Could you check a few things on this model? Use its own coordinates, in mm. Face numbers are marked on the shaded views. Coordinates: 2 decimals unless noted, no trailing zeros. Loops run counter-clockwise (first coordinate to the right, second up) from the corner with the lowest first, then second, coordinate; pieces in that order, holes last. Notation, with made-up numbers: (-21.5, 79) - (18.5, 79) arc R8 cw to (18.5, 89) - close; hole circle Ø5 at (88.25, 54.25). An arc over 180 degrees is marked (long way). Use CSV: the item, a comma, the result in double quotes.
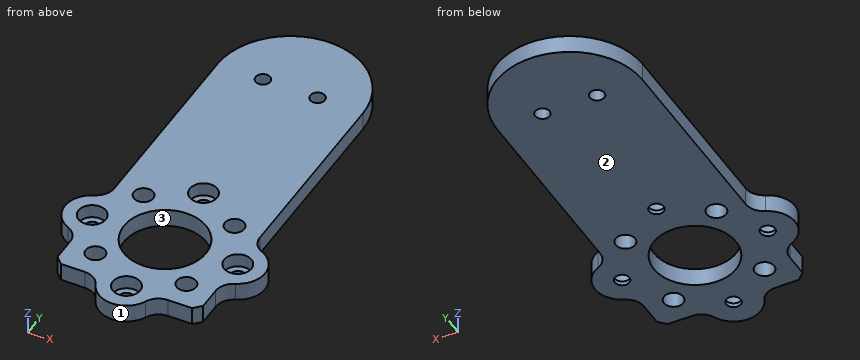
from build123d import *

# Parameters (mm, degrees)
SKETCH1_R                                       = 3.3782
SKETCH1_R_2                                     = 14.3129
BOSS_EXTRUDE1_DEPTH                             = 6.35
CBORE_FOR_10_SOCKET_HEAD_CAP_SCREW1_D           = 5.1054
CBORE_FOR_10_SOCKET_HEAD_CAP_SCREW1_CBORE_D     = 9.525
CBORE_FOR_10_SOCKET_HEAD_CAP_SCREW1_CBORE_DEPTH = 4.826
F_1_4_20_TAPPED_HOLE2_D                         = 5.1054
FILLET1_R                                       = 6.35
CHAMFER1_SIZE                                   = 2.54


with BuildPart() as part:
    # Sketch1 → Boss-Extrude1 (new body)
    with BuildSketch(Plane.XY):
        with BuildLine():
            Line((0, 0), (15.875, 0))
            ThreePointArc((15.875, 0), (25.4, -9.525), (34.925, 0))
            Line((34.925, 0), (50.8, 0))
            Line((50.8, 0), (50.8, 15.875))
            ThreePointArc((50.8, 15.875), (60.325, 25.4), (50.8, 34.925))
            Line((50.8, 34.925), (50.8, 107.95))
            ThreePointArc((50.8, 107.95), (25.4, 133.35), (0, 107.95))
            Line((0, 107.95), (0, 34.925))
            ThreePointArc((0, 34.925), (-9.525, 25.4), (0, 15.875))
            Line((0, 15.875), (0, 0))
        make_face()
        with Locations((41.275, 9.525)):
            Circle(SKETCH1_R, mode=Mode.SUBTRACT)
        with Locations((9.525, 9.525)):
            Circle(SKETCH1_R, mode=Mode.SUBTRACT)
        with Locations((9.525, 41.275)):
            Circle(SKETCH1_R, mode=Mode.SUBTRACT)
        with Locations((41.275, 41.275)):
            Circle(SKETCH1_R, mode=Mode.SUBTRACT)
        with Locations((25.4, 25.4)):
            Circle(SKETCH1_R_2, mode=Mode.SUBTRACT)
    extrude(amount=BOSS_EXTRUDE1_DEPTH)

    # CBORE for #10 Socket Head Cap Screw1 (through all)
    with Locations(Plane.XY.offset(6.35)):
        with Locations((0, 25.4), (50.8, 25.4), (25.4, 0), (25.4, 50.8)):
            CounterBoreHole(CBORE_FOR_10_SOCKET_HEAD_CAP_SCREW1_D / 2, CBORE_FOR_10_SOCKET_HEAD_CAP_SCREW1_CBORE_D / 2, CBORE_FOR_10_SOCKET_HEAD_CAP_SCREW1_CBORE_DEPTH)

    # 1/4-20 Tapped Hole2 (through all)
    with Locations(Plane(origin=(0, 0, 0), x_dir=(1, 0, 0), z_dir=(0, 0, -1))):
        with Locations((15.875, -107.95), (34.925, -107.95)):
            Hole(F_1_4_20_TAPPED_HOLE2_D / 2)

    # Fillet1
    fillet1_edges = [part.edges().sort_by_distance(p)[0] for p in [
        (0, 15.875, 3.175),
        (0, 34.925, 3.175),
        (50.8, 34.925, 3.175),
        (50.8, 15.875, 3.175),
        (34.925, 0, 3.175),
        (15.875, 0, 3.175),
    ]]
    fillet(fillet1_edges, radius=FILLET1_R)

    # Chamfer1
    chamfer1_edges = [part.edges().sort_by_distance(p)[0] for p in [
        (50.8, 0, 3.175),
        (0, 0, 3.175),
    ]]
    chamfer(chamfer1_edges, length=CHAMFER1_SIZE)


solid = part.part
(1) Thinking about a two-plate mould opening in X: for the marked faces 1, 2 and 3, which applies, +X half, -X half, draft (parallel to the pull), parting line (faces both ways), or undercut?
Computed:
face 1,"parting line"
face 2,"draft"
face 3,"undercut"
(2) Suppose I cut it at A-A (y = 25.4). State how many separate pieces and enclosed holes the cut face has, plus the area to 3 significant figures.
Computed:
separate pieces,"4"
enclosed holes,"0"
area,"154 mm²"
(3) Will these pins go through, and if not, where does the flat tip stop? pin 1 (1 mm diameter, centred on x = 49.5, z = 4, fed in from -Y); pin 2 (1 mm diameter, centred on x = 26.5, z = 2.5, fed in from -Y); pin 3 (3 mm diameter, centred on x = 21.5, z = 1.5, fed in from -Y).
Computed:
pin 1,"stops at y = 0.74"
pin 2,"stops at y = -9.51"
pin 3,"stops at y = -9.22"
(4) Suppose I cut it at D-D (y = 72.5). Write out the boundary of the cut face in (x, z), plus the area to 3 significant figures.
Computed:
outline,"(0, 0) - (50.8, 0) - (50.8, 6.35) - (0, 6.35) - close"
area,"323 mm²"
(5) Suppose I cut it at B-B (y = 50.8). Write out the boundary of the cut face in (x, z), plus the area to 3 significant figures.
Computed:
outline,"(0, 0) - (22.85, 0) - (22.85, 1.52) - (20.64, 1.52) - (20.64, 6.35) - (0, 6.35) - close; (27.95, 0) - (50.8, 0) - (50.8, 6.35) - (30.16, 6.35) - (30.16, 1.52) - (27.95, 1.52) - close"
area,"269 mm²"
(6) Please list where these lines run through material, in increasing order: line 1 (X direction, y = 107.95, z = 4.75); line 2 (Y direction, x = 41.5, z = 6.25); line 3 (Y direction, x = 11, z = 5.25).
Computed:
line 1,"x = 0 to 13.32, 18.43 to 32.37, 37.48 to 50.8"
line 2,"y = 0 to 6.15, 12.9 to 37.9, 44.65 to 127.6"
line 3,"y = 0 to 6.49, 12.56 to 38.24, 44.31 to 128.87"
